```python
from build123d import *

# Parameters (mm, degrees)
F0_R     = 1.75
F1_DEPTH = 4
F2_DEPTH = 24
F3_R     = 3.5
F4_R     = 1.5
F5_R     = 2


with BuildPart() as f1:
    # F0 (on Top) → F1 (new body)
    with BuildSketch(Plane.XY):
        with BuildLine():
            Line((-26, 0), (0, 0))
            Line((0, 0), (0, 25))
            Line((0, 25), (-22.5, 25))
            ThreePointArc((-22.5, 25), (-24.974874, 23.974874), (-26, 21.5))
            Line((-26, 21.5), (-26, 0))
        make_face()
        with Locations((-13, 12.5)):
            Circle(F0_R, mode=Mode.SUBTRACT)
        with BuildLine():
            Line((0, -25), (0, 0))
            Line((0, 0), (-26, 0))
            Line((-26, 0), (-26, -21.5))
            ThreePointArc((-26, -21.5), (-24.974874, -23.974874), (-22.5, -25))
            Line((-22.5, -25), (0, -25))
        make_face()
        with Locations((-13, -12.5)):
            Circle(F0_R, mode=Mode.SUBTRACT)
    extrude(amount=F1_DEPTH)

    # F0 (on Top) → F2 (join)
    with BuildSketch(Plane.XY):
        Polygon((0, 25), (0, 0), (0, -25), (4, -25), (4, 25), align=None)
    extrude(amount=F2_DEPTH)

    # F3
    f3_edges = [f1.edges().sort_by_distance(p)[0] for p in [
        (2, 25, 24),
        (2, -25, 24),
    ]]
    fillet(f3_edges, radius=F3_R)

    # F4
    f4_edges = [f1.edges().sort_by_distance(p)[0] for p in [
        (-24.974874, 23.974874, 0),
        (-26, 0, 0),
        (-24.974874, -23.974874, 0),
        (-9.25, -25, 0),
        (4, 0, 0),
        (-9.25, 25, 0),
        (-14.75, 12.5, 0),
        (-14.75, -12.5, 0),
        (4, -25, 10.25),
        (4, -23.974874, 22.974874),
        (4, 0, 24),
        (4, 25, 10.25),
        (4, 23.974874, 22.974874),
    ]]
    fillet(f4_edges, radius=F4_R)

    # F5
    f5_edges = [f1.edges().sort_by_distance(p)[0] for p in [
        (0, 0, 24),
        (0, -25, 12.25),
        (0, 25, 12.25),
    ]]
    fillet(f5_edges, radius=F5_R)


solid = f1.part
```
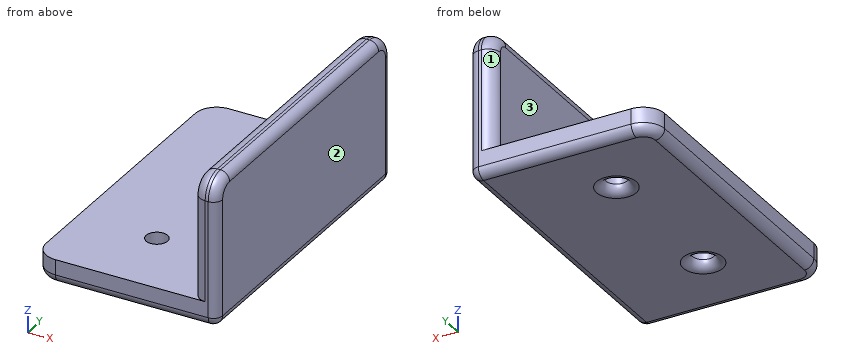
The listing builds one solid part. Answer for the finished solid, in the listing's coordinates (mm). Face numbers are marked on the shaded views. A direction names the side the tool comes from. Coordinates: 2 decimals unless noted, no trailing zeros. Write each loop counter-clockwise with the first axis right and the second up, starting at its lowest first coordinate (ties: lowest second). Pieces come first, ordered by that corner, then holes. Notation, with made-up numbers: (-18, 1.25) - (7, 1.25) arc R12 ccw to (7, 18.25) - close; hole circle Ø5 at (33.25, 44). An arc over 180 degrees is marked (long way). One line per item, written item: value.
1) Find section C-C (z = 14.75). Give the vertices of the cut face in (x, y), and give its area (3 significant figures).
Geometry check:
outline: (0, -23) arc R2 ccw to (2, -25) - (2.5, -25) arc R1.5 ccw to (4, -23.5) - (4, 23.5) arc R1.5 ccw to (2.5, 25) - (2, 25) arc R2 ccw to (0, 23) - close
area: 197 mm2
2) A tool of negligible diameter and unlimited length cuts with its end or side. For the marked faces 1, 2 and 3, from which of +Z, -Z, +X, -X, +Y, -Y can it reach the whole face along a straight path? Write none if from no direction.
Geometry check:
face 1: +Z, -X, +Y
face 2: +Z, -Z, +X, +Y, -Y
face 3: +Z, -X, +Y, -Y
3) Each of these flat-tipped pins is pushed along its axis until it touches: pin 1 Ø6 at (x, y) = (-10, -10) entering from +Z; pin 2 Ø12 at (x, z) = (-8.5, 13) entering from -Y (1 decimal); pin 3 Ø4 at (y, z) = (14, 6.5) entering from -X. Where does it stop, or does it pass through?
Geometry check:
pin 1: stops at z = 4
pin 2: passes through
pin 3: stops at x = 0
4) Find section B-B (y = 12.5). Give the vertices of the cut face in (x, z), and give its area (3 significant figures).
Geometry check:
outline: (-26, 1.5) arc R1.5 ccw to (-24.5, 0) - (-16.25, 0) arc R1.5 ccw to (-14.75, 1.5) - (-14.75, 4) - (-26, 4) - close; (-11.25, 1.5) arc R1.5 ccw to (-9.75, 0) - (2.5, 0) arc R1.5 ccw to (4, 1.5) - (4, 22.5) arc R1.5 ccw to (2.5, 24) - (2, 24) arc R2 ccw to (0, 22) - (0, 4) - (-11.25, 4) - close
area: 183 mm2
5) Find section A-A (x = -13). Give the vertices of the cut face in (y, z).
Geometry check:
outline: (-25, 1.5) arc R1.5 ccw to (-23.5, 0) - (-15.75, 0) arc R1.5 ccw to (-14.25, 1.5) - (-14.25, 4) - (-25, 4) - close; (-10.75, 1.5) arc R1.5 ccw to (-9.25, 0) - (9.25, 0) arc R1.5 ccw to (10.75, 1.5) - (10.75, 4) - (-10.75, 4) - close; (14.25, 1.5) arc R1.5 ccw to (15.75, 0) - (23.5, 0) arc R1.5 ccw to (25, 1.5) - (25, 4) - (14.25, 4) - close
6) Consider line 1 along Y through (x, z) = (-13, 2.3); line 2 along Z through (x, y) = (-20.5, 10). Determine where each line is inside the solid, lowest interval first. Write a range as from..to.
Geometry check:
line 1: y = -25..-14.25, -10.75..10.75, 14.25..25
line 2: z = 0..4
